from build123d import *

# Parameters (mm, degrees)
SKETCH1_R           = 7.5
EXTRUSION1_DEPTH    = 160
SKETCH2_R           = 2.25
EXTRUSION2_DEPTH    = 80
SKETCH4_R           = 9.988310786
EXTRUSION4_DEPTH    = 45
SKETCH5_R           = 7.5
SKETCH5_R_2         = 4
EXTRUSION5_DEPTH    = 15
SKETCH6_R           = 13.00139778
CUT_EXTRUDE1_DEPTH  = 45
SKETCH7_R           = 4.639288825
SKETCH7_R_2         = 2.05
BOSS_EXTRUDE1_DEPTH = 70


with BuildPart() as part:
    # Sketch1 → Extrusion1 (new body)
    with BuildSketch(Plane(origin=(0, 0, 0), x_dir=(-1, 0, 0), z_dir=(0, 1, 0))):
        with Locations(Location((0, 0, 0), (0, 0, 90))):
            Circle(SKETCH1_R)
    extrude(amount=EXTRUSION1_DEPTH)

    # Sketch2 → Extrusion2 (cut)
    with BuildSketch(Plane(origin=(0, 160, 0), x_dir=(-1, 0, 0), z_dir=(0, 1, 0))):
        with Locations(Location((0, 0, 0), (0, 0, 90))):
            Circle(SKETCH2_R)
    extrude(amount=-EXTRUSION2_DEPTH, mode=Mode.SUBTRACT)

    # Sketch4 → Extrusion4 (cut)
    with BuildSketch(Plane.XZ):
        Circle(SKETCH4_R)
    extrude(amount=-EXTRUSION4_DEPTH, mode=Mode.SUBTRACT)

    # Sketch5 → Extrusion5 (cut)
    with BuildSketch(Plane.XZ.offset(-45)):
        with Locations(Location((0, 0, 0), (0, 0, 270))):
            Circle(SKETCH5_R)
        with Locations(Location((0, 0, 0), (0, 0, 270))):
            Circle(SKETCH5_R_2, mode=Mode.SUBTRACT)
    extrude(amount=-EXTRUSION5_DEPTH, mode=Mode.SUBTRACT)

    # Sketch6 → Cut-Extrude1 (cut)
    with BuildSketch(Plane.XZ.offset(-45)):
        Circle(SKETCH6_R)
    extrude(amount=-CUT_EXTRUDE1_DEPTH, mode=Mode.SUBTRACT)

    # Sketch7 → Boss-Extrude1 (add)
    with BuildSketch(Plane.XZ.offset(-90)):
        Circle(SKETCH7_R)
        with Locations(Location((0, 0, 0), (0, 0, 270))):
            Circle(SKETCH7_R_2, mode=Mode.SUBTRACT)
    extrude(amount=-BOSS_EXTRUDE1_DEPTH)


solid = part.part
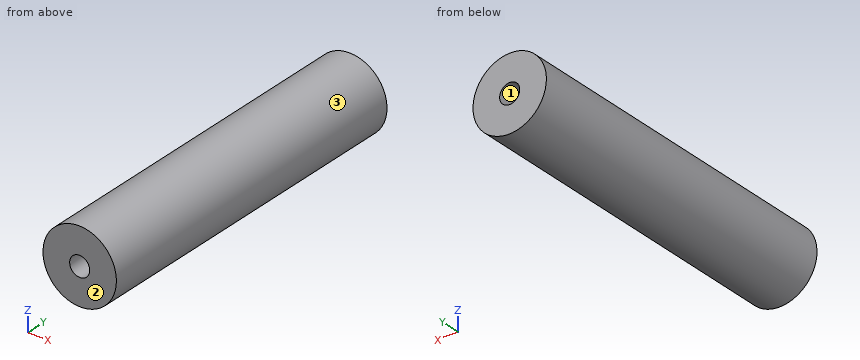
Verification items for the finished model (mm, model axes). Face numbers are marked on the shaded views. Give positions to 0.01 mm unless a question says otherwise; leave off trailing zeros. Write each loop counter-clockwise with the first axis right and the second up, starting at its lowest first coordinate (ties: lowest second). Pieces come first, ordered by that corner, then holes. Notation, with made-up numbers: M 70.5,34.5 L 110.5,34.5 A26 ccw 110.5,68.5 Z; hole C 60.5,-39 d1. An arc over 180 degrees is marked long. Write item = value, one per line.
(1) Material ranges on line 1 (X direction, y = 125.5, z = 0); line 2 (Z direction, x = 1.5, y = 107.5); line 3 (X direction, y = 134, z = 4), recorded low to high.
Found:
line_1 = -7.5 to -2.05, 2.05 to 7.5
line_2 = -7.35 to -1.4, 1.4 to 7.35
line_3 = -6.34 to 6.34
(2) Go/stop test with flat-tipped pins: pin 1 Ø8 at (x, y) = (5.5, 123.5) entering from -Z; pin 2 Ø4 at (y, z) = (102, -4) entering from +X; pin 3 Ø5 at (x, y) = (3.5, 111.5) entering from -Z. Record where each tip stops, or that it passes through.
Found:
pin_1 = -7.35
pin_2 = 7.23
pin_3 = -7.43
(3) Sectioned sample at B-B (z = 0). Record the cut outline in (x, y), then the cut area to 3 significant figures.
Found:
outline = M -7.5,90 L -2.05,90 L -2.05,160 L -7.5,160 Z; M 2.05,90 L 7.5,90 L 7.5,160 L 2.05,160 Z
area = 763 mm2
(4) Sectioned sample at A-A (x = 0). Record the cut outline in (y, z).
Found:
outline = M 90,-7.5 L 160,-7.5 L 160,-2.05 L 90,-2.05 Z; M 90,2.05 L 160,2.05 L 160,7.5 L 90,7.5 Z
(5) Draft check along Z on the marked faces 1, 2 and 3. Enter one of: released by +Z, released by -Z, zero draft, split by the parting line, or undercut.
Found:
face_1 = undercut
face_2 = zero draft
face_3 = split by the parting line
(6) Sectioned sample at D-D (z = -6). Record the cut outline in (x, y).
Found:
outline = M -4.5,90 L 4.5,90 L 4.5,160 L -4.5,160 Z
(7) Sectioned sample at C-C (y = 115.5). Record the cut outline in (x, z).
Found:
outline = C 0,0 d15; hole C 0,0 d4.1
